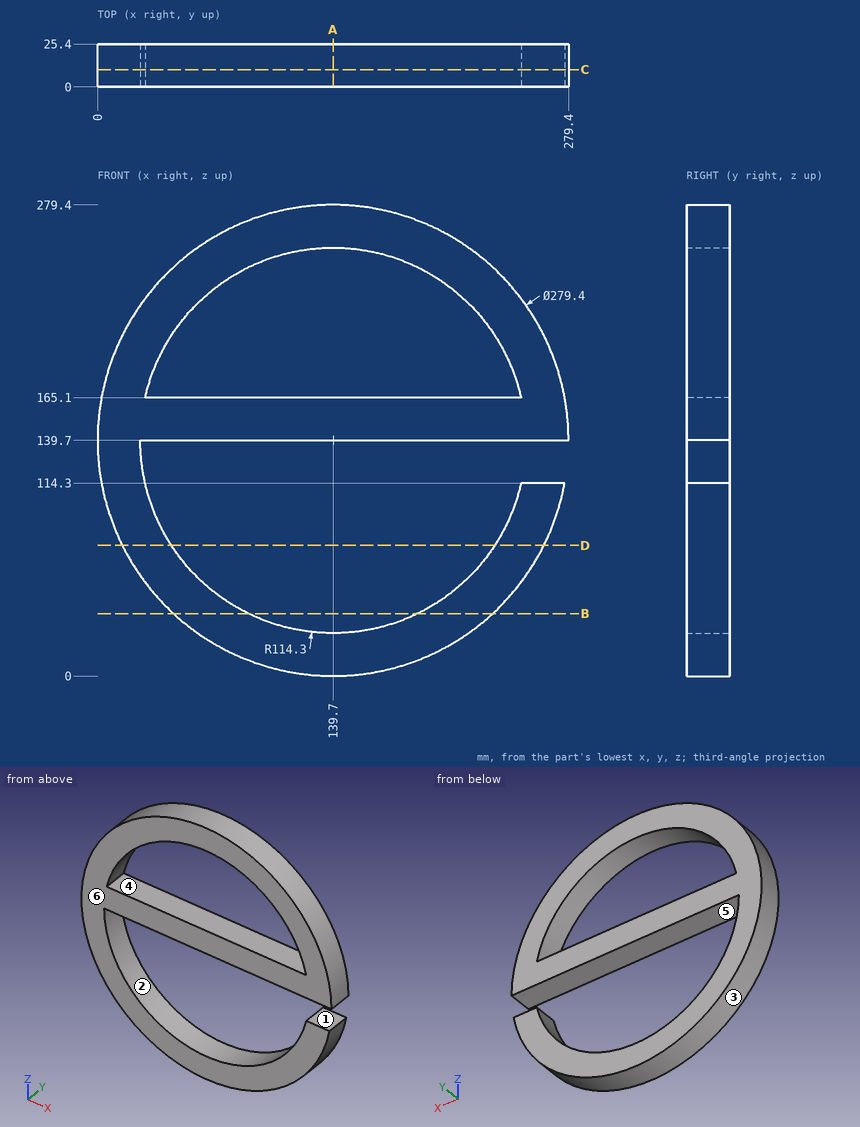
Source: three-view drawing plus pictorial views. Frame: mm from the lowest corner of the part. A direction names the side the tool comes from. Give positions to 0.01 mm unless a question says otherwise; leave off trailing zeros. Loops run counter-clockwise (first coordinate to the right, second up) from the corner with the lowest first, then second, coordinate; pieces in that order, holes last. Notation, with made-up numbers: M 27.5,-7 L 46.5,-7 A17 ccw 46.5,26 Z; hole C 23.5,46.25 d6. An arc over 180 degrees is marked long. Use CSV: the item, a comma, the result in double quotes.
(1) Section C-C, the plane y = 10.25. Return loops of the section in (x, z).
Outcome:
outline,"M 25.4,139.7 L 279.4,139.7 A139.7 ccw long 277.07,114.3 L 251.14,114.3 A114.3 cw Z; hole M 28.26,165.1 L 251.14,165.1 A114.3 ccw Z"
(2) Pin query (flat end, axial travel): P1, Ø5, axis at y = 19, z = 207.5, coming from the -X side; P2, Ø4, axis at x = 190.5, y = 18, coming from the -Z side; P3, Ø1.5, axis at x = 133.5, y = 11, coming from the +Z side; P4, Ø10, axis at x = 211.5, z = 40.5, coming from the -Y side. Return the tip coordinate at first contact, or that it passes through.
Outcome:
P1,"stops at x = 16.2"
P2,"stops at z = 8.8"
P3,"stops at z = 279.29"
P4,"stops at y = 0"
(3) Material intervals for L1, parallel to Z at x = 212, y = 8.5; L2, parallel to Z at x = 100, y = 4.75; L3, parallel to X at y = 6.5, z = 111.5, sorted ascending. Write a range as [from, to].
Outcome:
L1,"z = [20.16, 51.17], [139.7, 165.1], [228.23, 259.24]"
L2,"z = [5.76, 32.52], [139.7, 165.1], [246.88, 273.64]"
L3,"x = [2.88, 28.93], [250.47, 276.52]"
(4) Section D-D, the plane z = 77.5. Return loops of the section in (x, y), plus the area to 3 significant figures.
Outcome:
outline,"M 14.61,0 L 43.81,0 L 43.81,25.4 L 14.61,25.4 Z; M 235.59,0 L 264.79,0 L 264.79,25.4 L 235.59,25.4 Z"
area,"1,480 mm²"
(5) Section A-A, the plane x = 139.7. Return loops of the section in (y, z), plus the area to 3 significant figures.
Outcome:
outline,"M 0,0 L 25.4,0 L 25.4,25.4 L 0,25.4 Z; M 0,139.7 L 25.4,139.7 L 25.4,165.1 L 0,165.1 Z; M 0,254 L 25.4,254 L 25.4,279.4 L 0,279.4 Z"
area,"1,940 mm²"
(6) Pull-direction query (X, two-part tool) for the marked faces 1, 2 and 3; classes: pulls with the +X half, pulls with the -X half, needs draft (parallel to the pull), parting line crosses it, or undercut.
Outcome:
face 1,"needs draft"
face 2,"undercut"
face 3,"parting line crosses it"
(7) Section B-B, the plane z = 37. Return loops of the section in (x, y), plus the area to 3 significant figures.
Outcome:
outline,"M 45,0 L 89.53,0 L 89.53,25.4 L 45,25.4 Z; M 189.87,0 L 234.4,0 L 234.4,25.4 L 189.87,25.4 Z"
area,"2,260 mm²"
(8) Set-up query: the marked faces 4, 5 and 6. Return all of +Z, -Z, +X, -X, +Y, -Y with unobstructed straight access to the full face (end or side cutting, diameter ignored); none if empty.
Outcome:
face 4,"+Y, -Y"
face 5,"+X, +Y, -Y"
face 6,"+Z, -Z, +X, -X, -Y"
